```python
from build123d import *

# Parameters (mm, degrees)
F0_W             = 944
F0_H             = 1000
F1_DEPTH         = 550
F4_DEPTH         = 10
F4_COPIES2_COUNT = 2


# Not quite as in the source:
# - a pattern or mirror of a feature is missing from the dataset's text; its kind, count and spacing are read off the source's solid


with BuildPart() as f1:
    # F0 (on Front) → F1 (new body, symmetric)
    with BuildSketch(Plane.XZ):
        Rectangle(F0_W, F0_H)
    extrude(amount=F1_DEPTH, both=True)

    # F3 (on offset) → F4 (join, symmetric)
    with BuildSketch(Plane.XZ.offset(485)):
        Polygon((538, 470), (472, 470), (472, 302), (538, 302), (538, 370), (521, 370), (521, 322), (489, 322), (489, 450), (521, 450), (521, 402), (538, 402), align=None)
    f4 = extrude(amount=F4_DEPTH, both=True)

    # F4_copies: F4 across plane
    add(f4.mirror(Plane.ZX))

    # F4_copies1: F4 across plane
    add(f4.mirror(Plane(origin=(0, 0, 0), x_dir=(0, 0, -1), z_dir=(-1, 0, 0))))

    # F4_copies2: F4 ×2 about axis
    f4_copies2_axis = Axis((0, 0, 0), (0, 0, 1))
    for i in range(1, F4_COPIES2_COUNT):
        add(f4.rotate(f4_copies2_axis, i * 360 / F4_COPIES2_COUNT))


solid = f1.part
```
Source: CAD feature listing. Evaluate the final solid. Frame: model axes, mm. A direction names the side the tool comes from. Coordinates: 2 decimals unless noted, no trailing zeros. Loops run counter-clockwise (first coordinate to the right, second up) from the corner with the lowest first, then second, coordinate; pieces in that order, holes last. Notation, with made-up numbers: M 23.25,-16 L 32.25,-16 A18 cw 32.25,3 Z; hole C -22,35 d11. An arc over 180 degrees is marked long. Put each result on its own line as item: value. Start each with the question number.
1) Cut plane A-A on z = 55.5. Return the cut outline in (x, y), then the cut area to 3 significant figures.
2) Contact query for flat-ended pins moving along their axis: pin 1 Ø8.5 at (x, y) = (-525.5, -486.5) entering from +Z; pin 2 Ø2 at (y, z) = (100.5, -386) entering from +X; pin 3 Ø10 at (x, y) = (-495, 487.5) entering from -Z. Output: stop coordinate, or through.
3) Reachability of faces 1 (the face through (483, -495, 387)), 2 (the face through (483, 475, 387)), 3 (the face through (-483, -475, 387)), 4 (the face through (483, 495, 387)) from +Z, -Z, +X, -X, +Y, -Y: full face, straight path, thin tool, end or side. Return the list, or none.
4) Ray query, L1, parallel to X at y = -372, z = -112.5. Return the intervals inside material, ascending. Write a range as from..to.
5) Pull-direction query (Y, two-part tool) for faces 5 (the face through (-483, 475, 387)), 6 (the face through (-7, -550, 7)), 7 (the face through (-483, 495, 387)); classes: pulls with the +Y half, pulls with the -Y half, needs draft (parallel to the pull), parting line crosses it, or undercut.
6) Cut plane B-B on y = 205.5. Return the cut outline in (x, z), then the cut area to 3 significant figures.
The answers:
1. outline: M -472,-550 L 472,-550 L 472,550 L -472,550 Z
1. area: 1,040,000 mm²
2. pin 1: stops at z = 470
2. pin 2: stops at x = 472
2. pin 3: stops at z = 302
3. face 1: +Z, -Z, +X, -Y
3. face 2: +Z, -Z, +X
3. face 3: +Z, -Z, -X
3. face 4: +Z, -Z, +X, +Y
4. L1: x = -472..472
5. face 5: undercut
5. face 6: pulls with the -Y half
5. face 7: pulls with the +Y half
6. outline: M -472,-500 L 472,-500 L 472,500 L -472,500 Z
6. area: 944,000 mm²
